from build123d import *

# Parameters (mm, degrees)
SKETCH_1_W                  = 15
SKETCH_1_H                  = 16
EXTRUDE_1_DEPTH             = 13.5
SKETCH_2_W                  = 1
SKETCH_2_H                  = 16
CUT_EXTRUDE_2_DEPTH         = 7.5
SKETCH_4_W                  = 3.5
SKETCH_4_H                  = 5
CUT_EXTRUDE_4_DEPTH         = 15
SKETCH_5_W                  = 3.5
SKETCH_5_H                  = 3.5
CUT_EXTRUDE_9_DEPTH         = 6
CUT_EXTRUDE_10_REACH        = 13
SKETCH_6_W                  = 2.5
SKETCH_6_H                  = 1
SKETCH_7_W                  = 1
SKETCH_7_H                  = 2.5
CUT_EXTRUDE_11_DEPTH        = 11.5
SKETCH_8_W                  = 8
SKETCH_8_H                  = 1
CUT_EXTRUDE_12_DEPTH        = 17
HOLE_WIZARD_M31_AT_2_COUNT  = 2
HOLE_WIZARD_M31_AT_2_PITCH  = 10
HOLE_WIZARD_M31_AT_3_COUNT  = 2
HOLE_WIZARD_M31_AT_3_PITCH  = 7.071067812
HOLE_WIZARD_M31_AT_4_COUNT  = 2
HOLE_WIZARD_M31_AT_4_PITCH  = 7.071067812
HOLE_WIZARD_M33_D           = 2.5
HOLE_WIZARD_M33_DEPTH       = 7.5
HOLE_WIZARD_M33_CSINK_D     = 3.3
HOLE_WIZARD_M33_CSINK_ANGLE = 110
HOLE_WIZARD_M33_TIP         = 0.751075774
SKETCH_11_W                 = 7.5
SKETCH_11_H                 = 3.5
HOLE_WIZARD_M35_D           = 2.5
HOLE_WIZARD_M35_DEPTH       = 7.5
HOLE_WIZARD_M35_CSINK_D     = 3.3
HOLE_WIZARD_M35_CSINK_ANGLE = 110
HOLE_WIZARD_M35_TIP         = 0.751075774


with BuildPart() as part:
    # Эскиз1 → Вытянуть1 (new body)
    with BuildSketch(Plane.XY):
        Rectangle(SKETCH_1_W, SKETCH_1_H)
    extrude(amount=EXTRUDE_1_DEPTH)

    # Эскиз2 → Вырез-Вытянуть2 (cut)
    with BuildSketch(Plane(origin=(0, 0, 0), x_dir=(-1, 0, 0), z_dir=(0, 0, -1))):
        with Locations((7, 0)):
            Rectangle(SKETCH_2_W, SKETCH_2_H)
        with Locations((-7, 0)):
            Rectangle(SKETCH_2_W, SKETCH_2_H)
    extrude(amount=-CUT_EXTRUDE_2_DEPTH, mode=Mode.SUBTRACT)

    # Эскиз4 → Вырез-Вытянуть4 (cut, through all)
    with BuildSketch(Plane.ZY.offset(6.5)):
        with Locations((5.75, 5.5)):
            Rectangle(SKETCH_4_W, SKETCH_4_H)
        with Locations((5.75, -5.5)):
            Rectangle(SKETCH_4_W, SKETCH_4_H)
    extrude(amount=-CUT_EXTRUDE_4_DEPTH, mode=Mode.SUBTRACT)

    # Эскиз5 → Вырез-Вытянуть9 (cut)
    with BuildSketch(Plane(origin=(0, 3, 0), x_dir=(-1, 0, 0), z_dir=(0, 1, 0))):
        with Locations((-4.75, 5.75)):
            Rectangle(SKETCH_5_W, SKETCH_5_H)
        with Locations((4.75, 5.75)):
            Rectangle(SKETCH_5_W, SKETCH_5_H)
    extrude(amount=-CUT_EXTRUDE_9_DEPTH, mode=Mode.SUBTRACT)

    # Эскиз6 → Вырез-Вытянуть10 (cut, up to next)
    with BuildSketch(Plane(origin=(0, 3, 0), x_dir=(-1, 0, 0), z_dir=(0, 1, 0)), mode=Mode.PRIVATE) as cut_extrude_10_sk1:
        with Locations((-1.75, 7)):
            Rectangle(SKETCH_6_W, SKETCH_6_H)
    cut_extrude_10_tool1 = extrude(cut_extrude_10_sk1.sketch, amount=-CUT_EXTRUDE_10_REACH, mode=Mode.PRIVATE) & part.part
    add(cut_extrude_10_tool1.solids().sort_by_distance((1.75, 3, 7))[0], mode=Mode.SUBTRACT)
    # Эскиз6 → Вырез-Вытянуть10 (cut, up to next)
    with BuildSketch(Plane(origin=(0, 3, 0), x_dir=(-1, 0, 0), z_dir=(0, 1, 0)), mode=Mode.PRIVATE) as cut_extrude_10_sk2:
        with Locations((1.75, 7)):
            Rectangle(SKETCH_6_W, SKETCH_6_H)
    cut_extrude_10_tool2 = extrude(cut_extrude_10_sk2.sketch, amount=-CUT_EXTRUDE_10_REACH, mode=Mode.PRIVATE) & part.part
    add(cut_extrude_10_tool2.solids().sort_by_distance((-1.75, 3, 7))[0], mode=Mode.SUBTRACT)

    # Эскиз7 → Вырез-Вытянуть11 (cut, through all)
    with BuildSketch(Plane(origin=(3, 0, 0), x_dir=(0, 0, -1), z_dir=(1, 0, 0))):
        with Locations((-4.5, 1.75)):
            Rectangle(SKETCH_7_W, SKETCH_7_H)
        with Locations((-4.5, -1.75)):
            Rectangle(SKETCH_7_W, SKETCH_7_H)
    extrude(amount=-CUT_EXTRUDE_11_DEPTH, mode=Mode.SUBTRACT)

    # Эскиз8 → Вырез-Вытянуть12 (cut, through all)
    with BuildSketch(Plane(origin=(0, 8, 0), x_dir=(-1, 0, 0), z_dir=(0, 1, 0))):
        with Locations((1, 0.5)):
            Rectangle(SKETCH_8_W, SKETCH_8_H)
    extrude(amount=-CUT_EXTRUDE_12_DEPTH, mode=Mode.SUBTRACT)

    # Эскиз9 → Отверстие обработанное метчиком M31 (revolve, cut)
    with BuildSketch(Plane(origin=(0, -5, 13.5), x_dir=(0, -1, 0), z_dir=(1, 0, 0))):
        Polygon((0, 0), (0, 6), (1.75, 6), (1.25, 5.5), (1.25, 0.5), (1.75, 0), align=None)
    hole_wizard_m31 = revolve(axis=Axis((0, -5, 19.85), (0, 0, -1)), mode=Mode.SUBTRACT)

    # Отверстие обработанное метчиком M31 at 2: Отверстие обработанное метчиком M31 ×2
    with Locations(*[(0, i * HOLE_WIZARD_M31_AT_2_PITCH, 0) for i in range(1, HOLE_WIZARD_M31_AT_2_COUNT)]):
        add(hole_wizard_m31, mode=Mode.SUBTRACT)

    # Отверстие обработанное метчиком M31 at 3: Отверстие обработанное метчиком M31 ×2
    with Locations(*[Vector(0.707106781, 0.707106781, 0) * (i * HOLE_WIZARD_M31_AT_3_PITCH) for i in range(1, HOLE_WIZARD_M31_AT_3_COUNT)]):
        add(hole_wizard_m31, mode=Mode.SUBTRACT)

    # Отверстие обработанное метчиком M31 at 4: Отверстие обработанное метчиком M31 ×2
    with Locations(*[Vector(-0.707106781, 0.707106781, 0) * (i * HOLE_WIZARD_M31_AT_4_PITCH) for i in range(1, HOLE_WIZARD_M31_AT_4_COUNT)]):
        add(hole_wizard_m31, mode=Mode.SUBTRACT)

    # Отверстие обработанное метчиком M33
    with Locations(Plane(origin=(-7.5, 5, 10.5), x_dir=(0, 0, -1), z_dir=(-1, 0, 0))):
        with Locations((0, 0), (0, 10)):
            CounterSinkHole(HOLE_WIZARD_M33_D / 2, HOLE_WIZARD_M33_CSINK_D / 2, depth=HOLE_WIZARD_M33_DEPTH, counter_sink_angle=HOLE_WIZARD_M33_CSINK_ANGLE)
            with Locations((0, 0, -(HOLE_WIZARD_M33_DEPTH + HOLE_WIZARD_M33_TIP / 2))):  # 118° drill point
                Cone(0, HOLE_WIZARD_M33_D / 2, HOLE_WIZARD_M33_TIP, mode=Mode.SUBTRACT)

    # Эскиз11 → Вырез-Повернуть1 (revolve, cut)
    with BuildSketch(Plane(origin=(0, 0, 0), x_dir=(1, 0, 0), z_dir=(0, 1, 0))):
        with Locations((6.75, -5.75)):
            Rectangle(SKETCH_11_W, SKETCH_11_H)
    revolve(axis=Axis((0, 0, 0), (0, 0, 1)), mode=Mode.SUBTRACT)

    # Отверстие обработанное метчиком M35
    with Locations(Plane(origin=(7.5, 6.867633096, -0.651107824), x_dir=(0, 0, -1), z_dir=(1, 0, 0))):
        with Locations((-11.151107824, -1.867633096), (-11.151107824, -11.867633096)):
            CounterSinkHole(HOLE_WIZARD_M35_D / 2, HOLE_WIZARD_M35_CSINK_D / 2, depth=HOLE_WIZARD_M35_DEPTH, counter_sink_angle=HOLE_WIZARD_M35_CSINK_ANGLE)
            with Locations((0, 0, -(HOLE_WIZARD_M35_DEPTH + HOLE_WIZARD_M35_TIP / 2))):  # 118° drill point
                Cone(0, HOLE_WIZARD_M35_D / 2, HOLE_WIZARD_M35_TIP, mode=Mode.SUBTRACT)


solid = part.part
CAD build for the part. Positions are in the model's coordinates, mm. A direction names the side the tool comes from. Coordinates: 2 decimals unless noted, no trailing zeros. Write each loop counter-clockwise with the first axis right and the second up, starting at its lowest first coordinate (ties: lowest second). Pieces come first, ordered by that corner, then holes. Notation, with made-up numbers: (49.5, 15.5) - (60.5, 15.5) arc R32 ccw to (60.5, 49.5) - close; hole circle Ø3 at (34.25, 75.25). An arc over 180 degrees is marked (long way). Use a Markdown table: item, result. Add a question column.
Item 1: Band-saw the part on B-B, the plane y = -5. Give the number of separate pieces and of enclosed holes in the cut face, and give its area (3 significant figures).
Item 2: Drill centre lines: L1, parallel to Y at x = 0, z = 12.25; L2, parallel to Z at x = 2.75, y = -1; L3, parallel to Z at x = -4.25, y = -3.5. Where is each one in solid material? Low to high. Write a range as from..to.
Item 3: 3-axis set-ups, long thin cutter, end or side, ignore diameter. For faces 4 (the face through (1, 0, 6.5)), 5 (the face through (-4.36, -5.05, 9.25)), 6 (the face through (-6.5, 0, 2)): which of +Z, -Z, +X, -X, +Y, -Y reach the whole face in a straight line?
Item 4: Band-saw the part on A-A, the plane x = 5. Give the cut face in (y, z), and give its area (3 significant figures).
Item 5: Band-saw the part on C-C, the plane x = 2. Give the cut face in (y, z), and give its area (3 significant figures).
Item 6: Flat gauge pins, fed straight in: pin 1 (2 mm diameter, centred on y = 3.5, z = 2, fed in from +X); pin 2 (3 mm diameter, centred on y = 5, z = 10.5, fed in from +X); pin 3 (2 mm diameter, centred on y = -5, z = 10.5, fed in from -X); pin 4 (1.5 mm diameter, centred on y = 6, z = 2, fed in from -X). Where does each tip first touch, or does it go through?
Item 7: Mould opens along Y. For faces 1 (the face through (0, -0.5, 4.5)), 2 (the face through (-0.845, -4.079, 12.045)), 3 (the face through (0, 2, 4)) say: pulls with the +Y half, pulls with the -Y half, needs draft (parallel to the pull), parting line crosses it, or undercut.
Item 8: Band-saw the part on D-D, the plane y = 2.5. Give the cut face in (x, z).
Numbers:
| question | item | result |
|---|---|---|
| 1 | separate pieces | 5 |
| 1 | enclosed holes | 0 |
| 1 | area | 87.0 mm2 |
| 2 | L1 | -8..-6.25, -3.75..3.75, 6.25..8 |
| 2 | L2 | 1..4, 5..6.5, 7.5..13.5 |
| 2 | L3 | 1..4, 7.5..13.5 |
| 3 | face 4 | +X, +Y, -Y |
| 3 | face 5 | +X, -X |
| 3 | face 6 | -Z, -X, +Y, -Y |
| 4 | outline | (-8, 0) - (8, 0) - (8, 4) - (-8, 4) - close; (-8, 7.5) - (-1.75, 7.5) - (-1.25, 8) - (-1.25, 13) - (-1.75, 13.5) - (-8, 13.5) - close; (1.25, 8) - (1.75, 7.5) - (8, 7.5) - (8, 13.5) - (1.75, 13.5) - (1.25, 13) - close; hole circle Ø2.5 at (-5, 10.5); hole circle Ø2.5 at (5, 10.5) |
| 4 | area | 135 mm2 |
| 5 | outline | (-8, 1) - (8, 1) - (8, 4) - (0.5, 4) - (0.5, 5) - (2.24, 5) - (2.24, 6.5) - (-2.24, 6.5) - (-2.24, 5) - (-0.5, 5) - (-0.5, 4) - (-8, 4) - close; (-8, 7.5) - (8, 7.5) - (8, 13.5) - (-8, 13.5) - close; hole circle Ø2.5 at (-5, 10.5); hole circle Ø2.5 at (5, 10.5) |
| 5 | area | 142 mm2 |
| 6 | pin 1 | x = 6.5 |
| 6 | pin 2 | x = 7.39 |
| 6 | pin 3 | through |
| 6 | pin 4 | x = -6.5 |
| 7 | face 1 | pulls with the -Y half |
| 7 | face 2 | undercut |
| 7 | face 3 | needs draft |
| 8 | outline | (-7.5, 7.5) - (-0.5, 7.5) - (-0.5, 6.5) - (-1.66, 6.5) - (-1.66, 5) - (1.66, 5) - (1.66, 6.5) - (0.5, 6.5) - (0.5, 7.5) - (7.5, 7.5) - (7.5, 13.5) - (-7.5, 13.5) - close; (-6.5, 0) - (-5, 0) - (-5, 1) - (3, 1) - (3, 0) - (6.5, 0) - (6.5, 4) - (-6.5, 4) - close |
